from build123d import *

# Parameters (mm, degrees)
SKETCH3_R           = 5
BOSS_EXTRUDE1_DEPTH = 20


with BuildPart() as part:
    # Sketch2 → Revolve1 (revolve)
    with BuildSketch(Plane(origin=(0, 0, 0), x_dir=(0, 0, -1), z_dir=(1, 0, 0)), mode=Mode.PRIVATE) as revolve1_sk:
        Polygon((0, 0), (0, 4), (8, 4), (8, 6), (87, 6), (87, 8.5), (92, 8.5), (92, 4), (100, 4), (100, 0), align=None)
    revolve(revolve1_sk.sketch.rotate(Axis((0, 0, 0), (0, 0, -1)), 90), axis=Axis((0, 0, 0), (0, 0, -1)))

    # Sketch3 → Boss-Extrude1 (add)
    with BuildSketch(Plane(origin=(0, 0, -100), x_dir=(-1, 0, 0), z_dir=(0, 0, -1))):
        Circle(SKETCH3_R)
    extrude(amount=BOSS_EXTRUDE1_DEPTH)


solid = part.part
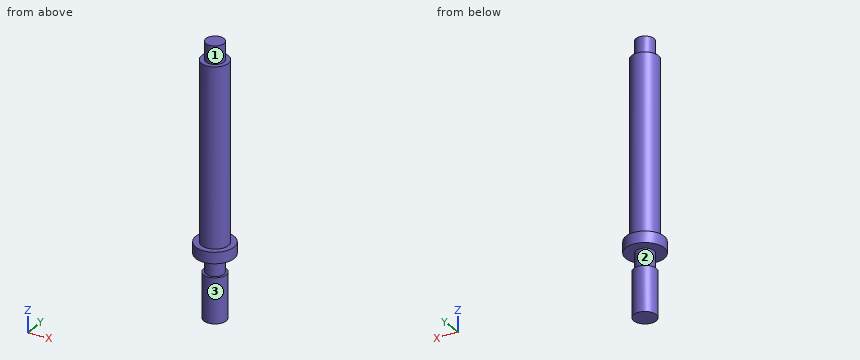
The listing builds one solid part. Answer for the finished solid, in the listing's coordinates (mm). Face numbers are marked on the shaded views. A direction names the side the tool comes from. Coordinates: 2 decimals unless noted, no trailing zeros. Order: outer loops, then holes, each group sorted by start corner. A loop starts at its lowest first (then second) coordinate and runs counter-clockwise, first axis right, second up. Notation, with made-up numbers: (7.25, 77.5) -> (46.25, 77.5) arc R14 cw to (46.25, 102.5) -> close; hole circle Ø4 at (67.25, 33.5). An arc over 180 degrees is marked (long way). Answer in a Markdown table with one row per item. Add a question column.
Item 1: Each of these flat-tipped pins is pushed along its axis until it touches: P1, Ø2, axis at x = 1, z = -13.5, coming from the -Y side; P2, Ø2, axis at x = 5, y = 4, coming from the +Z side; P3, Ø1, axis at x = -3, z = -81.5, coming from the +Y side. Where does it stop, or does it pass through?
Item 2: Find the intervals of material crossed by L1, parallel to Z at x = -1.75, y = -4; L2, parallel to Z at x = -6.5, y = -0.75; L3, parallel to X at y = -0.5, z = -34, in increasing order. Write a range as from..to.
Item 3: Find section C-C (z = -107.5). Write down the section's boundary in (x, y).
Item 4: Which of the six approach directions +Z, -Z, +X, -X, +Y, -Y give full straight-line access (tool end or side, diameter ignored) to the marked faces 1, 2 and 3?
Item 5: Find section D-D (y = 7.25). Write down the section's boundary in (x, z).
Item 6: Find section A-A (y = 0). Write down the section's boundary in (x, z), then the cut area to 3 significant figures.
Result set:
| question | item | result |
|---|---|---|
| 1 | P1 | stops at y = -6 |
| 1 | P2 | stops at z = -8 |
| 1 | P3 | stops at y = 5.45 |
| 2 | L1 | z = -120..-100, -92..-8 |
| 2 | L2 | z = -92..-87 |
| 2 | L3 | x = -5.98..5.98 |
| 3 | outline | circle Ø10 at (0, 0) |
| 4 | face 1 | +Z |
| 4 | face 2 | none |
| 4 | face 3 | -Z |
| 5 | outline | (-4.44, -92) -> (4.44, -92) -> (4.44, -87) -> (-4.44, -87) -> close |
| 6 | outline | (-8.5, -92) -> (-4, -92) -> (-4, -100) -> (-5, -100) -> (-5, -120) -> (5, -120) -> (5, -100) -> (4, -100) -> (4, -92) -> (8.5, -92) -> (8.5, -87) -> (6, -87) -> (6, -8) -> (4, -8) -> (4, 0) -> (-4, 0) -> (-4, -8) -> (-6, -8) -> (-6, -87) -> (-8.5, -87) -> close |
| 6 | area | 1,360 mm² |
